Check sheet for the modelled part. Datum: model origin and axes. Units: mm. Face numbers are marked on the shaded views. A direction names the side the tool comes from. Coordinates: 2 decimals unless noted, no trailing zeros. Loops run counter-clockwise (first coordinate to the right, second up) from the corner with the lowest first, then second, coordinate; pieces in that order, holes last. Notation, with made-up numbers: M 8,58.25 L 60,58.25 A14 cw 60,68.25 Z; hole C 3,9.5 d4. An arc over 180 degrees is marked long. Answer in a Markdown table with one row per item. Add a question column.
```python
from build123d import *

# Parameters (mm, degrees)
SKETCH1_R                = 11
BOSS_EXTRUDE1_DEPTH      = 3.7
SKETCH2_R                = 6.9
CUT_EXTRUDE1_DEPTH       = 3.7
BOSS_EXTRUDE2_DEPTH      = 0.1
BOSS_EXTRUDE2_DEPTH_BACK = 0.1
SKETCH3_R                = 8.700899362


with BuildPart() as part:
    # Sketch1 → Boss-Extrude1 (new body)
    with BuildSketch(Plane(origin=(0, 0, 0), x_dir=(1, 0, 0), z_dir=(0, 1, 0))):
        with Locations(Location((0, 0, 0), (0, 0, 270))):
            Circle(SKETCH1_R)
    extrude(amount=BOSS_EXTRUDE1_DEPTH)

    # Sketch2 → Cut-Extrude1 (cut)
    with BuildSketch(Plane(origin=(0, 3.7, 0), x_dir=(1, 0, 0), z_dir=(0, 1, 0))):
        with Locations(Location((0, 0, 0), (0, 0, 270))):
            Circle(SKETCH2_R)
    extrude(amount=-CUT_EXTRUDE1_DEPTH, mode=Mode.SUBTRACT)

    # Sketch3 → Boss-Extrude2 (add, two sides: drawn at the far end of the back side and taken through both)
    with BuildSketch(Plane(origin=(0, 1.85, 0), x_dir=(1, 0, 0), z_dir=(0, 1, 0)).offset(-BOSS_EXTRUDE2_DEPTH_BACK)):
        Circle(SKETCH3_R)
    extrude(amount=BOSS_EXTRUDE2_DEPTH + BOSS_EXTRUDE2_DEPTH_BACK)


solid = part.part
```
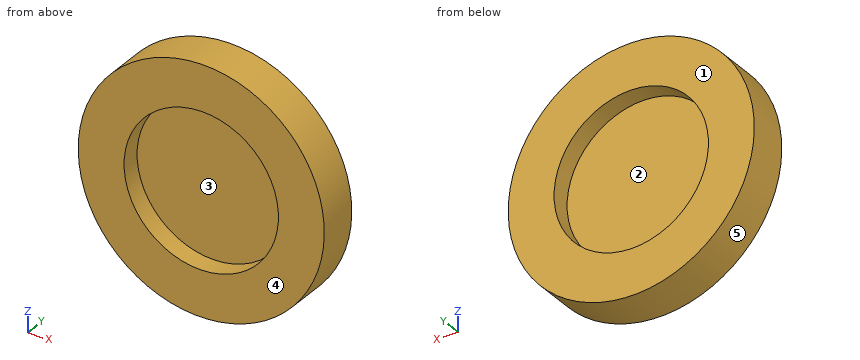
Q1. Cross-section at A-A (z = 0). Record the cut outline in (x, y).
Q2. Cross-section at B-B (x = 0). Record the cut outline in (y, z).
Q3. Cross-section at D-D (z = -8). Record the cut outline in (x, y), plus the area to 3 significant figures.
Q4. Thickness scan on L1, parallel to X at y = 2.3, z = 0; L2, parallel to X at y = 0.7, z = 6; L3, parallel to Z at x = -1.5, y = 2.25. Record the ranges inside material, lowest first.
Q5. Mould release check, pull along X, two halves, no side actions. Record for the marked faces 3, 4 and 5: released by +X, released by -X, zero draft, split by the parting line, or undercut.
Q6. Access from +Z, -Z, +X, -X, +Y, -Y to the whole of each face (thin tool, end or side, straight path). Record for the marked faces 1 and 2.
Q7. Go/stop test with flat-tipped pins: pin 1 (1.5 mm diameter, centred on y = 2, z = -3.5, fed in from +X); pin 2 (1.5 mm diameter, centred on y = 1, z = 2.5, fed in from +X); pin 3 (4 mm diameter, centred on x = -2, z = 0, fed in from +Y); pin 4 (11 mm diameter, centred on x = 1.5, z = 2, fed in from -Y). Record where each tip stops, or that it passes through.
Q8. Cross-section at C-C (y = 0.4). Record the cut outline in (x, z), plus the area to 3 significant figures.
Answer key:
| question | item | result |
|---|---|---|
| 1 | outline | M -11,0 L -6.9,0 L -6.9,1.75 L 6.9,1.75 L 6.9,0 L 11,0 L 11,3.7 L 6.9,3.7 L 6.9,1.95 L -6.9,1.95 L -6.9,3.7 L -11,3.7 Z |
| 2 | outline | M 0,-11 L 3.7,-11 L 3.7,-6.9 L 1.95,-6.9 L 1.95,6.9 L 3.7,6.9 L 3.7,11 L 0,11 L 0,6.9 L 1.75,6.9 L 1.75,-6.9 L 0,-6.9 Z |
| 3 | outline | M -7.55,0 L 7.55,0 L 7.55,3.7 L -7.55,3.7 Z |
| 3 | area | 55.9 mm^2 |
| 4 | L1 | -11 to -6.9, 6.9 to 11 |
| 4 | L2 | -9.22 to -3.41, 3.41 to 9.22 |
| 4 | L3 | -10.9 to -6.73, 6.73 to 10.9 |
| 5 | face 3 | undercut |
| 5 | face 4 | zero draft |
| 5 | face 5 | split by the parting line |
| 6 | face 1 | +Z, -Z, +X, -X, +Y |
| 6 | face 2 | +Y |
| 7 | pin 1 | x = 10.65 |
| 7 | pin 2 | x = 10.86 |
| 7 | pin 3 | y = 1.95 |
| 7 | pin 4 | y = 0 |
| 8 | outline | C 0,0 d22; hole C 0,0 d13.8 |
| 8 | area | 231 mm^2 |
